Source: CAD feature listing. Evaluate the final solid. Frame: model axes, mm. Face numbers are marked on the shaded views. A direction names the side the tool comes from. Round coordinates to 2 decimals unless told otherwise and drop trailing zeros. Loops run counter-clockwise (first coordinate to the right, second up) from the corner with the lowest first, then second, coordinate; pieces in that order, holes last.
(1) Section B-B, the plane x = 3.3. Return the cut outline in (y, z).
(2) Section A-A, the plane x = 0.7. Return the cut outline in (y, z), plus the area to 3 significant figures.
(3) Mould query, pull axis Y, two halves, no side actions, for the marked faces 1, 2 and 3. Classes: pulls with the +Y half, pulls with the -Y half, needs draft (parallel to the pull), parting line crosses it, or undercut.
(4) Set-up query: the marked faces 4 and 5. Return all of +Z, -Z, +X, -X, +Y, -Y with unobstructed straight access to the full face (end or side cutting, diameter ignored); none if empty.
(5) Material intervals for probe 1 along Z at (x, y) = (0.45, -0.65); probe 2 along Z at (x, y) = (2.9, 0.05); probe 3 along Z at (x, y) = (2.5, 0.45), sorted ascending.
(6) First-contact query: pin 1 Ø0.6 at (x, z) = (1, 0) entering from -Y; pin 2 Ø1 at (x, y) = (1.5, -1) entering from -Z. Flat tips, straight axial feed; report the tip coordinate or a pass-through.
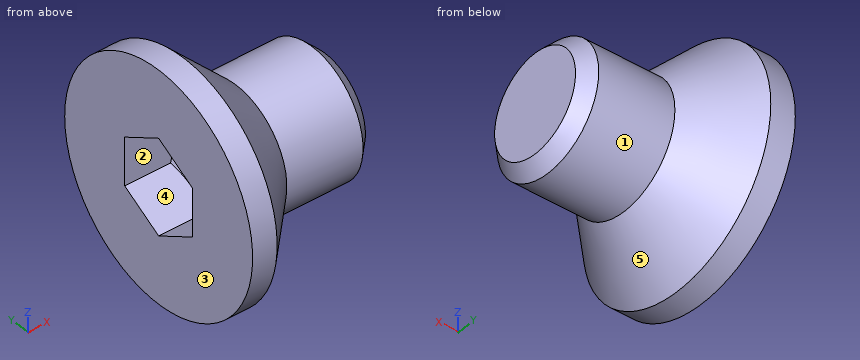
Autodesk Inventor part; units mm, degrees
ref_plane "Work Plane1" through (104.775, 0, 0) normal (0, 0, -1) x (1, 0, 0)
ref_plane "YZ Plane" through (0, 0, 0) normal (1, 0, 0) x (0, 1, 0)
ref_plane "XZ Plane" through (0, 0, 0) normal (0, 1, 0) x (-1, 0, 0)
sketch "Skizze1" plane through (0, 0, 0) normal (0, 0, 1) x (1, 0, 0)
  line L0 (8, 0) -> (8, 1.5)
  line L1 (8, 1.5) -> (3.36, 1.5)
  line L2 (3.36, 1.5) -> (3.0533, 1.5)
  line L3 (0, 2.77) -> (0, 1.1547)
  line L4 (0, 1.1547) -> (1.1, 1.1547)
  line L5 (1.1, 1.1547) -> (1.7667, 0)
  line L6 (1.7667, 0) -> (8, 0)
  line L7 (0, 2.77) -> (0.59, 2.77)
  line L8 (0.59, 2.77) -> (1.86, 1.5)
  line L9 (3.0533, 1.5) -> (1.86, 1.5)
  line L10 (3.36, 1.5) -> (1.86, 1.5) construction
  line L11 (1.86, 1.5) -> (1.86, 1.5)
  line L12 (-1.6, 0) -> (9.6, 0)
  line L13 (0, -0.554) -> (0, 3.324)
  dimension "d0" = 8
  dimension "d1" = 4.64
  dimension "d2" = 1.1
  dimension "d3" = 3
  dimension "d6" = 1.86
  dimension "d7" = 45
  dimension "d8" = 2.3094
  dimension "d9" = 60
  dimension "d10" = 5.54
  dimension "d11" = 3
  dimension "d12" = 0.3067
revolve "Körper" add sketch "Skizze1" angle 360 about axis through (1.7667, 0, 0) along (1, 0, 0) contours L6 L5 L4 L3 L7 L8 L9 L2 L1 L0
sketch "Skizze2" plane through (0, 0, 0) normal (-1, 0, 0) x (0, 0, 1)
  circle A0 centre (0, 0) radius 1.1547
  line L0 (0, -3.878) -> (0, 3.878)
  line L1 (-3.878, 0) -> (3.878, 0)
  line L2 (1.1547, 0) -> (0.5774, -1)
  line L3 (0.5774, -1) -> (-0.5774, -1)
  line L4 (-0.5774, -1) -> (-1.1547, 0)
  line L5 (-1.1547, 0) -> (-0.5774, 1)
  line L6 (-0.5774, 1) -> (0.5774, 1)
  line L7 (0.5774, 1) -> (1.1547, 0)
  point P0 (0, 1.1547)
extrude "Loch" add sketch "Skizze2" against normal up to next contours L7 A0 | A0 L2 | L6 L0 A0 | A0 L0 L3 | L0 L6 A0 | A0 L3 L0 | L4 A0 | A0 L5
thread "Gewinde"
ref_plane "Work Plane1" through (104.775, 0, 0) normal (0, 0, -1) x (1, 0, 0)
chamfer "Fase1" distance 0.3067 distance2 0.3067 1 edges at (8, -1.5, 0) measured on face at (8, -0.8298, -0.2045)
sketch "Skizze4" plane through (8, 0, 0) normal (1, 0, 0) x (0, 0, -1)
  circle A0 centre (0, 0) radius 1.5
extrude "Extrusion3" cut sketch "Skizze4" against normal blind 4
chamfer "Fasen3" distance 0.307 angle 45 1 edges at (4, -1.5, 0)
equation "\"d17\" = -0.5 * SPD + 0.5 * GD"
equation "\"d18\" = GUL"
equation "\"d0\" = NLG"
equation "\"d1\" = GEL"
equation "\"d2\" = INTI"
equation "\"d3\" = GD"
equation "\"d6\" = KOH"
equation "\"d7\" = 0.5 * SEWI"
equation "\"d8\" = 1.1547 * SW"
equation "\"d10\" = KOD"
equation "\"d11\" = BDM"
equation "\"d12\" = GAL"
equation "\"NLG\" = 8"
equation "\"INTI\" = 1.1"
equation "\"GEL\" = 4.64"
equation "\"GAL\" = 0.61345 * PTC"
equation "\"KOH\" = 1.86"
equation "\"KOD\" = 5.54"
equation "\"GUL\" = 0.61345 * PTC"
equation "\"SPD\" = NND - 1.2269 * PTC"
equation "\"BDM\" = NND"
equation "\"GD\" = NND"
equation "\"SEWI\" = 90deg"
equation "\"SW\" = 2"
equation "\"TOA\" = 30deg"
equation "\"GD1\" = THREADDIA - 1.2269 * PTC"
equation "\"EPV\" = 3.36"
equation "\"THREADDIA\" = 3"
equation "\"PTC\" = 0.5"
equation "\"NND\" = 3"
equation "\"E0\" = 2.31"
properties part number "ISO 10642  - M3  x  8" material "Stahl"
Output values:
1. outline: circle Ø3 at (0, 0)
2. outline: circle Ø5.32 at (0, 0); hole (-1, -0.58) - (0, -1.15) - (1, -0.58) - (1, 0.58) - (0, 1.15) - (-1, 0.58) - close
2. area: 18.8 mm2
3. face 1: parting line crosses it
3. face 2: undercut
3. face 3: needs draft
4. face 4: -X
4. face 5: +X
5. probe 1: z = -2.69 to -0.78, 0.78 to 2.69
5. probe 2: z = -1.5 to 1.5
5. probe 3: z = -1.43 to 1.43
6. pin 1: stops at y = -2.66
6. pin 2: stops at z = -2.18
